```python
from build123d import *

# Parameters (mm, degrees)
BOSS_EXTRUDE1_DEPTH                                 = 12.7
F_4_CLEARANCE_HOLE1_D                               = 3.3
F_4_CLEARANCE_HOLE1_DEPTH                           = 12.7
F_1_4_CLEARANCE_HOLE1_D                             = 6.6
F_1_4_CLEARANCE_HOLE1_DEPTH                         = 12.7
F_1_4_CLEARANCE_HOLE2_D                             = 6.8
F_1_4_CLEARANCE_HOLE2_DEPTH                         = 12.7
CSK_FOR_1_4_FLAT_HEAD_MACHINE_SCREW_100_D           = 6.6
CSK_FOR_1_4_FLAT_HEAD_MACHINE_SCREW_100_DEPTH       = 12.7
CSK_FOR_1_4_FLAT_HEAD_MACHINE_SCREW_100_CSINK_D     = 12.6
CSK_FOR_1_4_FLAT_HEAD_MACHINE_SCREW_100_CSINK_ANGLE = 90
F_10_CLEARANCE_HOLE1_D                              = 5
F_10_CLEARANCE_HOLE1_DEPTH                          = 15
F_10_CLEARANCE_HOLE2_D                              = 5
F_10_CLEARANCE_HOLE2_DEPTH                          = 10
F_1_3_4_CLEARANCE_HOLE1_D                           = 45
F_1_3_4_CLEARANCE_HOLE1_DEPTH                       = 5
F_1_4_CLEARANCE_HOLE3_D                             = 6.6
F_1_4_CLEARANCE_HOLE3_DEPTH                         = 12.7
CHAMFER1_SIZE                                       = 3


with BuildPart() as part:
    # Sketch1 → Boss-Extrude1 (new body)
    with BuildSketch(Plane(origin=(0, 0, 0), x_dir=(-1, 0, 0), z_dir=(0, 0, -1))):
        with BuildLine():
            Line((44.45, 0), (44.45, 60))
            Line((44.45, 60), (-44.45, 60))
            Line((-44.45, 60), (-44.45, 0))
            ThreePointArc((-44.45, 0), (0, -44.45), (44.45, 0))
        make_face()
    extrude(amount=-BOSS_EXTRUDE1_DEPTH)

    # #4 Clearance Hole1
    with Locations(Plane.XY.offset(12.7)):
        with Locations((26.35, 0), (0, -26.35), (-26.35, 0), (0, 26.35)):
            Hole(F_4_CLEARANCE_HOLE1_D / 2, depth=F_4_CLEARANCE_HOLE1_DEPTH)

    # 1/4 Clearance Hole1
    with Locations(Plane(origin=(0, 0, 0), x_dir=(-1, 0, 0), z_dir=(0, 0, -1))):
        with Locations((8.85, 30), (23.65, 38), (23.65, 22)):
            Hole(F_1_4_CLEARANCE_HOLE1_D / 2, depth=F_1_4_CLEARANCE_HOLE1_DEPTH)

    # 1/4 Clearance Hole2
    with Locations(Plane.XY.offset(12.7)):
        with Locations((11.472503772, 49.692873304)):
            Hole(F_1_4_CLEARANCE_HOLE2_D / 2, depth=F_1_4_CLEARANCE_HOLE2_DEPTH)

    # CSK for 1/4 Flat Head Machine Screw (100)1
    with Locations(Plane(origin=(0, 0, 0), x_dir=(-1, 0, 0), z_dir=(0, 0, -1))):
        with Locations((23.65, 54), (38.45, 6), (38.45, 30)):
            CounterSinkHole(CSK_FOR_1_4_FLAT_HEAD_MACHINE_SCREW_100_D / 2, CSK_FOR_1_4_FLAT_HEAD_MACHINE_SCREW_100_CSINK_D / 2, depth=CSK_FOR_1_4_FLAT_HEAD_MACHINE_SCREW_100_DEPTH, counter_sink_angle=CSK_FOR_1_4_FLAT_HEAD_MACHINE_SCREW_100_CSINK_ANGLE)

    # #10 Clearance Hole1
    with Locations(Plane(origin=(0, 60, 0), x_dir=(1, 0, 0), z_dir=(0, 1, 0))):
        with Locations((-38.45, -6.35), (-8.85, -6.35)):
            Hole(F_10_CLEARANCE_HOLE1_D / 2, depth=F_10_CLEARANCE_HOLE1_DEPTH)

    # #10 Clearance Hole2
    with Locations(Plane(origin=(44.45, 0, 0), x_dir=(0, 0, -1), z_dir=(1, 0, 0))):
        with Locations((-6.35, 7), (-6.35, 53), (-6.35, 30)):
            Hole(F_10_CLEARANCE_HOLE2_D / 2, depth=F_10_CLEARANCE_HOLE2_DEPTH)

    # 1-3/4 Clearance Hole1
    with Locations(Plane(origin=(0, 0, 0), x_dir=(-1, 0, 0), z_dir=(0, 0, -1))):
        with Locations((0, 0)):
            Hole(F_1_3_4_CLEARANCE_HOLE1_D / 2, depth=F_1_3_4_CLEARANCE_HOLE1_DEPTH)

    # 1/4 Clearance Hole3
    with Locations(Plane.XY.offset(12.7)):
        with Locations((12.374075778, 12.373661564), (17.499, -0.001), (12.372661564, -12.375075778), (-0.002, -17.5), (-12.376075778, -12.373661564), (-17.501, 0.001), (-12.374661564, 12.375075778), (0, 17.5)):
            Hole(F_1_4_CLEARANCE_HOLE3_D / 2, depth=F_1_4_CLEARANCE_HOLE3_DEPTH)

    # Chamfer1
    chamfer1_edges = [part.edges().sort_by_distance(p)[0] for p in [
        (-26.95, 22, 0),
        (-26.95, 38, 0),
        (-12.15, 30, 0),
    ]]
    chamfer(chamfer1_edges, length=CHAMFER1_SIZE)


solid = part.part
```
Verification items for the finished model (mm, model axes). A direction names the side the tool comes from. Give positions to 0.01 mm unless a question says otherwise; leave off trailing zeros. Write each loop counter-clockwise with the first axis right and the second up, starting at its lowest first coordinate (ties: lowest second). Pieces come first, ordered by that corner, then holes. Notation, with made-up numbers: (55, 50) - (87, 50) arc R35 cw to (87, 88) - close; hole circle Ø11 at (16.5, 39.25). An arc over 180 degrees is marked (long way). Put each result on its own line as item: value.
Q1. Scan lines: probe 1 along Y at (x, z) = (0, 9.5); probe 2 along X at (y, z) = (13.5, 12.25); probe 3 along Y at (x, z) = (-23.65, 7). Record each from-to range of solid material in increasing order. Write a range as from..to.
Result:
probe 1: -44.45..-28, -24.7..-20.8, -14.2..14.2, 20.8..24.7, 28..60
probe 2: -44.45..-15.48, -9.27..9.27, 15.48..44.45
probe 3: -37.64..18.7, 25.3..34.7, 41.3..50.7, 57.3..60
Q2. Depth check by flat-ended pin: P1, Ø8.5, axis at x = -38.45, y = 30, coming from the -Z side; P2, Ø3, axis at y = 30, z = 6.35, coming from the +X side; P3, Ø2.5, axis at x = -8, z = 7, coming from the +Y side. Enter the tip coordinate at first touch or a pass-through.
Result:
P1: z = 2.05
P2: x = 34.45
P3: y = 45
Q3. Set-up check for faces 4 (the face through (39.38, 31.69, 4.51)), 5 (the face through (-35.3, 6.99, 7.92)): record each of +Z, -Z, +X, -X, +Y, -Y from which the full face is reachable in a straight line by a thin tool's end or side.
Result:
face 4: +X
face 5: +Z, -Z
Q4. Section check D-D on x = -38.45. Record the cut outline in (y, z), and give its area (3 significant figures).
Result:
outline: (-22.3, 0) - (-0.3, 0) - (2.7, 3) - (2.7, 12.7) - (-22.3, 12.7) - close; (9.3, 3) - (12.3, 0) - (23.7, 0) - (26.7, 3) - (26.7, 12.7) - (9.3, 12.7) - close; (33.3, 3) - (36.3, 0) - (60, 0) - (60, 3.85) - (45, 3.85) - (45, 8.85) - (60, 8.85) - (60, 12.7) - (33.3, 12.7) - close
area: 785 mm2
Q5. Section check B-B on x = 17. Record the cut outline in (y, z).
Result:
outline: (-41.07, 0) - (-14.74, 0) - (-14.74, 5) - (-3.26, 5) - (-3.26, 12.7) - (-41.07, 12.7) - close; (3.26, 5) - (14.74, 5) - (14.74, 0) - (60, 0) - (60, 12.7) - (3.26, 12.7) - close
Q6. Mould release check, pull along Z, two halves, no side actions. Record for faces 1 (the face through (-9.597, 26.636, 2.854)), 2 (the face through (39.38, 5.479, 4.366)), 3 (the face through (-14.15, -9.59, 8.8)): released by +Z, released by -Z, zero draft, split by the parting line, or undercut.
Result:
face 1: released by -Z
face 2: undercut
face 3: zero draft
Q7. Section check C-C on z = 10.25. Count the separate pieces of the cut face and the enclosed holes in it, and give its area (3 significant figures).
Result:
separate pieces: 1
enclosed holes: 19
area: 7,890 mm2
Q8. Section check A-A on y = -26.35. Record the cut outline in (x, z).
Result:
outline: (-35.8, 0) - (-1.65, 0) - (-1.65, 12.7) - (-35.8, 12.7) - close; (1.65, 0) - (35.8, 0) - (35.8, 12.7) - (1.65, 12.7) - close
